from build123d import *

# Parameters (mm, degrees)
SKETCH1_W                      = 96
SKETCH1_H                      = 96
BOSS_EXTRUDE1_DEPTH            = 8
SKETCH2_W                      = 92
SKETCH2_H                      = 92
COMPONENT_PLATFORM_DEPTH       = 6
CABLE_SLOTS_DEPTH              = 6
SKETCH4_R                      = 7.5
CENTER_MASS_CUT_DEPTH          = 6
INNER_CORNER_FILLETS_R         = 3
M3X0_5_TAPPED_HOLE1_AT_2_COUNT = 2
M3X0_5_TAPPED_HOLE1_AT_2_PITCH = 70
M3X0_5_TAPPED_HOLE2_AT_2_COUNT = 2
M3X0_5_TAPPED_HOLE2_AT_2_PITCH = 70


with BuildPart() as part:
    # Sketch1 → Boss-Extrude1 (new body)
    with BuildSketch(Plane.XY):
        Rectangle(SKETCH1_W, SKETCH1_H)
    extrude(amount=BOSS_EXTRUDE1_DEPTH)

    # Sketch2 → Component Platform (cut)
    with BuildSketch(Plane.XY.offset(8)):
        Rectangle(SKETCH2_W, SKETCH2_H)
    extrude(amount=-COMPONENT_PLATFORM_DEPTH, mode=Mode.SUBTRACT)

    # Sketch3 → Cable Slots (cut, symmetric)
    with BuildSketch(Plane.XY.offset(2)):
        with BuildLine():
            Line((-33.878679656, -25.121320344), (-28.878679656, -20.121320344))
            ThreePointArc((-28.878679656, -20.121320344), (-28.228361402, -19.148050297), (-28, -18))
            Line((-28, -18), (-28, 18))
            ThreePointArc((-28, 18), (-28.228361402, 19.148050297), (-28.878679656, 20.121320344))
            Line((-28.878679656, 20.121320344), (-33.878679656, 25.121320344))
            ThreePointArc((-33.878679656, 25.121320344), (-34.851949703, 25.771638598), (-36, 26))
            Line((-36, 26), (-48, 26))
            Line((-48, 26), (-48, -26))
            Line((-48, -26), (-36, -26))
            ThreePointArc((-36, -26), (-34.851949703, -25.771638598), (-33.878679656, -25.121320344))
        make_face()
        with BuildLine():
            Line((48, -26), (48, 26))
            Line((48, 26), (36, 26))
            ThreePointArc((36, 26), (34.851949703, 25.771638598), (33.878679656, 25.121320344))
            Line((33.878679656, 25.121320344), (28.878679656, 20.121320344))
            ThreePointArc((28.878679656, 20.121320344), (28.228361402, 19.148050297), (28, 18))
            Line((28, 18), (28, -18))
            ThreePointArc((28, -18), (28.228361402, -19.148050297), (28.878679656, -20.121320344))
            Line((28.878679656, -20.121320344), (33.878679656, -25.121320344))
            ThreePointArc((33.878679656, -25.121320344), (34.851949703, -25.771638598), (36, -26))
            Line((36, -26), (48, -26))
        make_face()
    extrude(amount=CABLE_SLOTS_DEPTH, both=True, mode=Mode.SUBTRACT)

    # Sketch4 → Center Mass Cut (cut)
    with BuildSketch(Plane.XY.offset(2)):
        Circle(SKETCH4_R)
    extrude(amount=-CENTER_MASS_CUT_DEPTH, mode=Mode.SUBTRACT)

    # Inner Corner Fillets
    inner_corner_fillets_edges = [part.edges().sort_by_distance(p)[0] for p in [
        (-46, -46, 5),
        (-46, 46, 5),
        (46, 46, 5),
        (46, -46, 5),
    ]]
    fillet(inner_corner_fillets_edges, radius=INNER_CORNER_FILLETS_R)

    # Sketch10 → M3x0.5 Tapped Hole1 (revolve, cut)
    with BuildSketch(Plane(origin=(48, -35, 5), x_dir=(0, 0, -1), z_dir=(0, 1, 0))):
        Polygon((0, 0), (0, 10.751075774), (1.25, 10), (1.25, 0), align=None)
    m3x0_5_tapped_hole1 = revolve(axis=Axis((54.35, -35, 5), (-1, 0, 0)), mode=Mode.SUBTRACT)

    # M3x0.5 Tapped Hole1 at 2: M3x0.5 Tapped Hole1 ×2
    with Locations(*[(0, i * M3X0_5_TAPPED_HOLE1_AT_2_PITCH, 0) for i in range(1, M3X0_5_TAPPED_HOLE1_AT_2_COUNT)]):
        add(m3x0_5_tapped_hole1, mode=Mode.SUBTRACT)

    # Sketch13 → M3x0.5 Tapped Hole2 (revolve, cut)
    with BuildSketch(Plane(origin=(-35, -48, 5), x_dir=(0, 0, -1), z_dir=(1, 0, 0))):
        Polygon((0, 0), (0, 10.751075774), (1.25, 10), (1.25, 0), align=None)
    m3x0_5_tapped_hole2 = revolve(axis=Axis((-35, -54.35, 5), (0, 1, 0)), mode=Mode.SUBTRACT)

    # M3x0.5 Tapped Hole2 at 2: M3x0.5 Tapped Hole2 ×2
    with Locations(*[(i * M3X0_5_TAPPED_HOLE2_AT_2_PITCH, 0, 0) for i in range(1, M3X0_5_TAPPED_HOLE2_AT_2_COUNT)]):
        add(m3x0_5_tapped_hole2, mode=Mode.SUBTRACT)

    # Mirror1: M3x0.5 Tapped Hole1 across plane
    add(m3x0_5_tapped_hole1.mirror(Plane(origin=(0, 0, 0), x_dir=(0, 0, 1), z_dir=(1, 0, 0))), mode=Mode.SUBTRACT)

    # Mirror1 copy 1 sketch → Mirror1 copy 1 (revolve, cut)
    with BuildSketch(Plane(origin=(-48, 35, 5), x_dir=(0, 0, -1), z_dir=(0, 1, 0))):
        Polygon((0, 0), (0, -10.751075774), (1.25, -10), (1.25, 0), align=None)
    revolve(axis=Axis((-54.35, 35, 5), (-1, 0, 0)), mode=Mode.SUBTRACT)

    # Mirror2: M3x0.5 Tapped Hole2 across plane
    add(m3x0_5_tapped_hole2.mirror(Plane(origin=(0, 0, 0), x_dir=(0, 0, 1), z_dir=(0, -1, 0))), mode=Mode.SUBTRACT)

    # Mirror2 copy 1 sketch → Mirror2 copy 1 (revolve, cut)
    with BuildSketch(Plane(origin=(35, 48, 5), x_dir=(0, 0, -1), z_dir=(1, 0, 0))):
        Polygon((0, 0), (0, -10.751075774), (1.25, -10), (1.25, 0), align=None)
    revolve(axis=Axis((35, 54.35, 5), (0, 1, 0)), mode=Mode.SUBTRACT)


solid = part.part
Design review of the part built by this model. Coordinates are the model's own, in mm. A direction names the side the tool comes from. Round coordinates to 2 decimals unless told otherwise and drop trailing zeros. Order: outer loops, then holes, each group sorted by start corner. A loop starts at its lowest first (then second) coordinate and runs counter-clockwise, first axis right, second up. Notation, with made-up numbers: M -38.5,18.25 L -5.5,18.25 A19 cw -5.5,44.25 Z; hole C -27.5,61 d6. An arc over 180 degrees is marked long. Answer as CSV lines item,"result". Start each with the question number.
1) Add section A-A (x = -39). Give the boundary of the cut face in (y, z).
2) Tool access review of faces 1 (the face through (31.414, 22.656, 1.014)), 2 (the face through (-31.414, -22.656, 0.986)), 3 (the face through (-11, 1, 2)): name each direction out of +Z, -Z, +X, -X, +Y, -Y from which nothing blocks a thin tool from reaching the whole face with its end or side.
3) Wall thickness on line 1 along X through (y, z) = (-46.55, 5); line 2 along Y through (x, z) = (46.6, 5); line 3 along X through (y, z) = (-33.5, 7.75): over which ranges is each line inside the solid? List them lowest first. Write a range as [from, to].
4) Add section C-C (y = 0). Give the boundary of the cut face in (x, z).
5) For pin 1 Ø2 at (y, z) = (-35, 5) entering from +X; pin 2 Ø1.6 at (y, z) = (0.5, 1) entering from +X; pin 3 Ø8 at (x, y) = (9.5, -24) entering from +Z, all flat-tipped, find the tip position at first contact; note any pin that passes through.
6) Add section B-B (y = 35). Give the boundary of the cut face in (x, z).
7) The part is to be moulded in two halves that separate along Z. For faces 4 (the face through (33.76, -47.01, 5.16)), 5 (the face through (-45, -26, 1)), 6 (the face through (-11, 47, 8)), say which applies: +Z half, -Z half, draft (parallel to the pull), parting line (faces both ways), or undercut.
8) Add section D-D (x = 0). Give the boundary of the cut face in (y, z).
Resolved:
1,outline,"M -48,0 L -26,0 L -26,2 L -46,2 L -46,8 L -48,8 Z; M 26,0 L 48,0 L 48,8 L 46,8 L 46,2 L 26,2 Z"
2,face 1,"+Z, -Z, +X"
2,face 2,"+Z, -Z, -X"
2,face 3,"+Z"
3,line 1,"[-48, -36.25], [-33.75, 33.75], [36.25, 48]"
3,line 2,"[-48, -36.25], [-33.75, -26], [26, 33.75], [36.25, 48]"
3,line 3,"[-48, -46], [46, 48]"
4,outline,"M -28,0 L -7.5,0 L -7.5,2 L -28,2 Z; M 7.5,0 L 28,0 L 28,2 L 7.5,2 Z"
5,pin 1,"through"
5,pin 2,"x = 28"
5,pin 3,"z = 2"
6,outline,"M -48,0 L 48,0 L 48,3.75 L 46,3.75 L 46,2 L -46,2 L -46,3.75 L -48,3.75 Z; M -48,6.25 L -46,6.25 L -46,8 L -48,8 Z; M 46,6.25 L 48,6.25 L 48,8 L 46,8 Z"
7,face 4,"undercut"
7,face 5,"draft"
7,face 6,"+Z half"
8,outline,"M -48,0 L -7.5,0 L -7.5,2 L -46,2 L -46,8 L -48,8 Z; M 7.5,0 L 48,0 L 48,8 L 46,8 L 46,2 L 7.5,2 Z"
